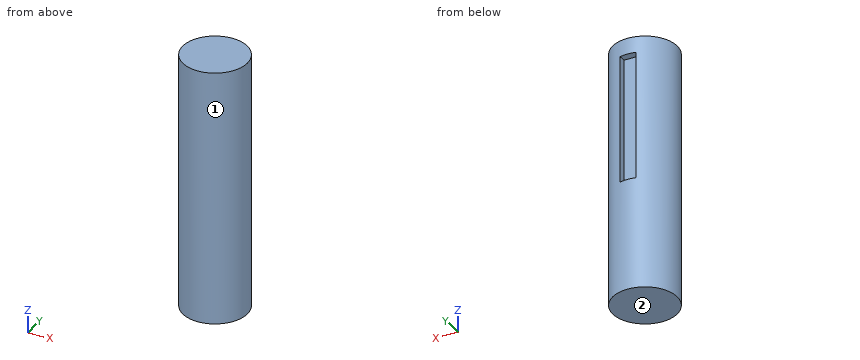
```python
from build123d import *

# Parameters (mm, degrees)
SKETCH1_R           = 10
BOSS_EXTRUDE1_DEPTH = 80
SKETCH3_W           = 5
SKETCH3_H           = 5
CUT_EXTRUDE1_DEPTH  = 40


with BuildPart() as part:
    # Sketch1 → Boss-Extrude1 (new body)
    with BuildSketch(Plane.XY):
        Circle(SKETCH1_R)
    extrude(amount=BOSS_EXTRUDE1_DEPTH)

    # Sketch3 → Cut-Extrude1 (cut)
    with BuildSketch(Plane(origin=(0, 0, 75), x_dir=(-1, 0, 0), z_dir=(0, 0, -1))):
        with Locations((0, 10)):
            Rectangle(SKETCH3_W, SKETCH3_H)
    extrude(amount=CUT_EXTRUDE1_DEPTH, mode=Mode.SUBTRACT)


solid = part.part
```
For this review, take the finished solid that the model builds, in its own axes (mm). Face numbers are marked on the shaded views. Round coordinates to 2 decimals unless told otherwise and drop trailing zeros. Write each loop counter-clockwise with the first axis right and the second up, starting at its lowest first coordinate (ties: lowest second). Pieces come first, ordered by that corner, then holes. Notation, with made-up numbers: (-14.5, 6.5) - (20.5, 6.5) arc R14 cw to (20.5, 26.5) - close; hole circle Ø9 at (5, -30). An arc over 180 degrees is marked (long way). Put each result on its own line as item: value.
Q1. Wall thickness on probe 1 along Y at (x, z) = (0.25, 28.5); probe 2 along X at (y, z) = (5, 27.5); probe 3 along X at (y, z) = (-0.75, 38): over which ranges is each line inside the solid? List them lowest first.
Solved:
probe 1: y = -10 to 10
probe 2: x = -8.66 to 8.66
probe 3: x = -9.97 to 9.97
Q2. We need section D-D (z = 22). Give the boundary of the cut face in (x, y), and give its area (3 significant figures).
Solved:
outline: circle Ø20 at (0, 0)
area: 314 mm2
Q3. Insertion check: pin 1 Ø3 at (x, z) = (2, 42) entering from +Y; pin 2 Ø2.5 at (y, z) = (8, 63.5) entering from -X; pin 3 Ø8 at (x, z) = (6, 11.5) entering from +Y. Each pin has a flat end and moves straight along its axis. Give the tip position at first contact, or say it passes through.
Solved:
pin 1: stops at y = 9.68
pin 2: stops at x = -7.38
pin 3: stops at y = 9.8
Q4. Mouldability with a two-part tool opening along X and no side actions: class the marked faces 1 and 2 as released by +X, released by -X, zero draft, split by the parting line, or undercut.
Solved:
face 1: split by the parting line
face 2: zero draft
Q5. We need section C-C (y = -2). Give the boundary of the cut face in (x, z).
Solved:
outline: (-9.8, 0) - (9.8, 0) - (9.8, 80) - (-9.8, 80) - close
Q6. We need section B-B (z = 69). Give the boundary of the cut face in (x, y).
Solved:
outline: (-2.5, 7.5) - (-2.5, 9.68) arc R10 ccw (long way) to (2.5, 9.68) - (2.5, 7.5) - close
Q7. We need section A-A (x = 0). Give the boundary of the cut face in (y, z), and give its area (3 significant figures).
Solved:
outline: (-10, 0) - (10, 0) - (10, 35) - (7.5, 35) - (7.5, 75) - (10, 75) - (10, 80) - (-10, 80) - close
area: 1,500 mm2
